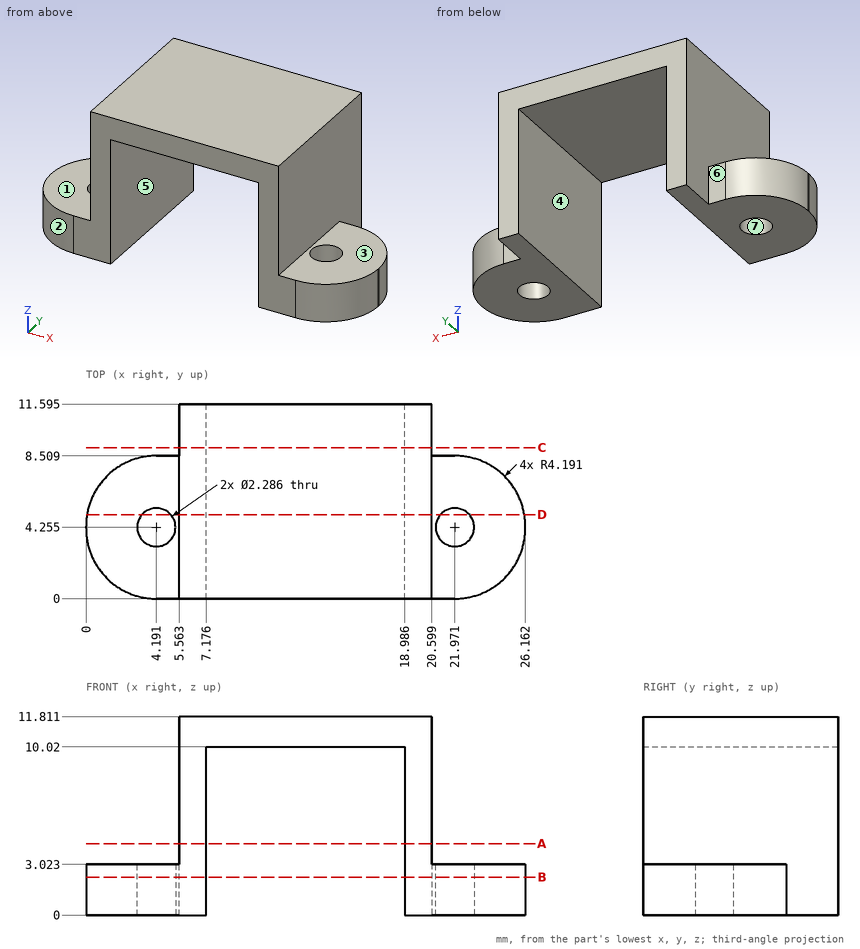
Geometry check sheet. Reference: drawing and pictorial views, mm from the part's lowest x, y, z. A direction names the side the tool comes from. Round coordinates to 2 decimals unless told otherwise and drop trailing zeros. Loops run counter-clockwise (first coordinate to the right, second up) from the corner with the lowest first, then second, coordinate; pieces in that order, holes last. Notation, with made-up numbers: (-17.5, 87) - (29.5, 87) arc R23 ccw to (29.5, 115) - close; hole circle Ø7 at (-26, 10.5). An arc over 180 degrees is marked (long way). Use a Markdown table: item, result.
Q1. Draft check along Y on the marked faces 5, 6 and 7. Enter one of: released by +Y, released by -Y, zero draft, split by the parting line, or undercut.
Solutions:
| item | result |
|---|---|
| face 5 | zero draft |
| face 6 | released by +Y |
| face 7 | undercut |
Q2. Material ranges on line 1 (X direction, y = 3.5, z = 6) (1 decimal); line 2 (Z direction, x = 4.5, y = 6); line 3 (X direction, y = 2.5, z = 1.25) (1 decimal), recorded low to high.
Solutions:
| item | result |
|---|---|
| line 1 | x = 5.6 to 7.2, 19 to 20.6 |
| line 2 | z = 0 to 3.02 |
| line 3 | x = 0.4 to 7.2, 19 to 25.8 |
Q3. Cross-section at D-D on y = 5. Record the cut outline in (x, z) (1 decimal).
Solutions:
| item | result |
|---|---|
| outline | (0.1, 0) - (3.3, 0) - (3.3, 3) - (0.1, 3) - close; (5.1, 0) - (7.2, 0) - (7.2, 10) - (19, 10) - (19, 0) - (21.1, 0) - (21.1, 3) - (20.6, 3) - (20.6, 11.8) - (5.6, 11.8) - (5.6, 3) - (5.1, 3) - close; (22.8, 0) - (26.1, 0) - (26.1, 3) - (22.8, 3) - close |
Q4. Cross-section at C-C on y = 9. Record the cut outline in (x, z) (1 decimal).
Solutions:
| item | result |
|---|---|
| outline | (5.6, 0) - (7.2, 0) - (7.2, 10) - (19, 10) - (19, 0) - (20.6, 0) - (20.6, 11.8) - (5.6, 11.8) - close |
Q5. Cross-section at A-A on z = 4.25. Record the cut outline in (x, y) (1 decimal).
Solutions:
| item | result |
|---|---|
| outline | (5.6, 0) - (7.2, 0) - (7.2, 11.6) - (5.6, 11.6) - close; (19, 0) - (20.6, 0) - (20.6, 11.6) - (19, 11.6) - close |
Q6. Go/stop test with flat-tipped pins: P1, Ø0.7, axis at x = 21, z = 1, coming from the +Y side; P2, Ø1.7, axis at x = 23.5, y = 6, coming from the +Z side; P3, Ø6, axis at x = 6.5, y = 6, coming from the -Z side; P4, Ø6, axis at x = 15, y = 3.5, coming from the -Z side. Record where each tip stops, or that it passes through.
Solutions:
| item | result |
|---|---|
| P1 | stops at y = 8.51 |
| P2 | stops at z = 3.02 |
| P3 | stops at z = 0 |
| P4 | stops at z = 10.02 |
Q7. Access from +Z, -Z, +X, -X, +Y, -Y to the whole of each face (thin tool, end or side, straight path). Record for the marked faces 1, 2, 3 and 4.
Solutions:
| item | result |
|---|---|
| face 1 | +Z, -X, +Y, -Y |
| face 2 | +Z, -Z, -X, -Y |
| face 3 | +Z, +X, +Y, -Y |
| face 4 | -Z, +Y, -Y |
Q8. Cross-section at B-B on z = 2.25. State how many separate pieces and enclosed holes the cut face has, plus the area to 3 significant figures.
Solutions:
| item | result |
|---|---|
| separate pieces | 2 |
| enclosed holes | 2 |
| area | 109 mm2 |
